```python
from build123d import *

# Parameters (mm, degrees)
ESTRUSIONE_ESTRUSIONE1_DEPTH = 15
SCHIZZO3_W                   = 33
SCHIZZO3_H                   = 6
TAGLIO_ESTRUSIONE1_DEPTH     = 127.609636284
TAGLIO_ESTRUSIONE2_DEPTH     = 127.609636284
FORO_15_0_15_2_D             = 15
FORO_12_0_12_1_D             = 12
SMUSSO1_SIZE                 = 2


with BuildPart() as part:
    # Schizzo2 → Estrusione-Estrusione1 (new, symmetric)
    with BuildSketch(Plane.XY):
        Polygon((0, 0), (123, 0), (123, 13), (115, 13), (115, 26), (30, 26), (30, 20), (0, 20), align=None)
    extrude(amount=ESTRUSIONE_ESTRUSIONE1_DEPTH, both=True)

    # Schizzo3 → Taglio-Estrusione1 (cut, through all)
    with BuildSketch(Plane(origin=(0, 26, 0), x_dir=(1, 0, 0), z_dir=(0, 1, 0))):
        with Locations((106.5, -12)):
            Rectangle(SCHIZZO3_W, SCHIZZO3_H)
        with Locations((106.5, 12)):
            Rectangle(SCHIZZO3_W, SCHIZZO3_H)
    extrude(amount=-TAGLIO_ESTRUSIONE1_DEPTH, mode=Mode.SUBTRACT)

    # Schizzo4 → Taglio-Estrusione2 (cut, through all)
    with BuildSketch(Plane(origin=(0, 26, 0), x_dir=(1, 0, 0), z_dir=(0, 1, 0))):
        with BuildLine():
            Line((45, 5), (75, 5))
            ThreePointArc((75, 5), (80, 0), (75, -5))
            Line((75, -5), (45, -5))
            ThreePointArc((45, -5), (40, 0), (45, 5))
        make_face()
    extrude(amount=-TAGLIO_ESTRUSIONE2_DEPTH, mode=Mode.SUBTRACT)

    # Foro Ø15.0 (15)-2 (through all)
    with Locations(Plane(origin=(0, 20, 0), x_dir=(1, 0, 0), z_dir=(0, 1, 0))):
        with Locations((15, 0)):
            Hole(FORO_15_0_15_2_D / 2)

    # Foro Ø12.0 (12)-1 (through all)
    with Locations(Plane.XY.offset(9)):
        with Locations((102, 12)):
            Hole(FORO_12_0_12_1_D / 2)

    # Smusso1
    smusso1_edges = [part.edges().sort_by_distance(p)[0] for p in [
        (0, 10, -15),
        (0, 10, 15),
    ]]
    chamfer(smusso1_edges, length=SMUSSO1_SIZE)


solid = part.part
```
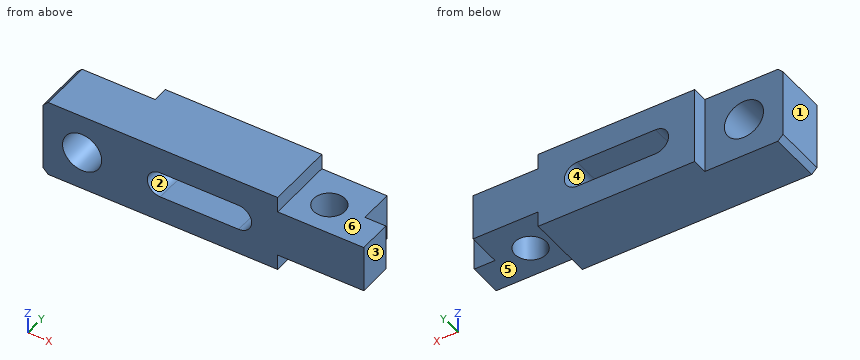
CAD build for the part. Positions are in the model's coordinates, mm. Face numbers are marked on the shaded views. A direction names the side the tool comes from. Round coordinates to 2 decimals unless told otherwise and drop trailing zeros. Order: outer loops, then holes, each group sorted by start corner. A loop starts at its lowest first (then second) coordinate and runs counter-clockwise, first axis right, second up. Notation, with made-up numbers: (82.25, -24.75) - (99.25, -24.75) arc R21 ccw to (99.25, -11.75) - close; hole circle Ø4 at (48, -32.5). An arc over 180 degrees is marked (long way). Answer in a Markdown table with one row per item. Add a question column.
(1) Band-saw the part on B-B on x = 102. List the corners of the cut face in (y, z), and give its area (3 significant figures).
(2) Mould opens along X. For the marked faces 1, 2 and 3 say: +X half, -X half, draft (parallel to the pull), parting line (faces both ways), or undercut.
(3) Band-saw the part on C-C on y = 4.25. List the corners of the cut face in (x, z), and give its area (3 significant figures).
(4) 3-axis set-ups, long thin cutter, end or side, ignore diameter. For the marked faces 4, 5 and 6: which of +Z, -Z, +X, -X, +Y, -Y reach the whole face in a straight line?
(5) Drop flat-ended pins along their axis: pin 1 Ø6.5 at (y, z) = (16.5, -11.5) entering from +X; pin 2 Ø3 at (x, y) = (104.5, 8) entering from +Z; pin 3 Ø2.5 at (x, z) = (118, 2.5) entering from +Y. Give the stop position or say it passes through.
(6) Probe L1, parallel to Y at x = 102, z = -2; L2, parallel to Z at x = 50.5, y = 13; L3, parallel to Z at x = 15, y = 12.25. List the from-to ranges inside material, lowest first. Write a range as [from, to].
(7) Band-saw the part on A-A on z = 0. List the corners of the cut face in (x, y), and give its area (3 significant figures).
(8) Band-saw the part on D-D on x = 62.5. List the corners of the cut face in (y, z), and give its area (3 significant figures).
Data:
| question | item | result |
|---|---|---|
| 1 | outline | (0, -9) - (6, -9) - (6, 9) - (0, 9) - close; (18, -9) - (26, -9) - (26, 9) - (18, 9) - close |
| 1 | area | 252 mm^2 |
| 2 | face 1 | -X half |
| 2 | face 2 | undercut |
| 2 | face 3 | +X half |
| 3 | outline | (0, -13) - (2, -15) - (90, -15) - (90, -9) - (123, -9) - (123, 9) - (90, 9) - (90, 15) - (2, 15) - (0, 13) - close; hole circle Ø15 at (15, 0); hole (45, -5) - (75, -5) arc R5 ccw to (75, 5) - (45, 5) arc R5 ccw to start |
| 3 | area | 2,730 mm^2 |
| 4 | face 4 | +Y, -Y |
| 4 | face 5 | -Z, +X, +Y, -Y |
| 4 | face 6 | +Z, +X, +Y, -Y |
| 5 | pin 1 | stops at x = 115 |
| 5 | pin 2 | stops at z = 9 |
| 5 | pin 3 | stops at y = 13 |
| 6 | L1 | y = [0, 6], [18, 26] |
| 6 | L2 | z = [-15, -5], [5, 15] |
| 6 | L3 | z = [-15, -7.5], [7.5, 15] |
| 7 | outline | (0, 0) - (7.5, 0) - (7.5, 20) - (0, 20) - close; (22.5, 0) - (40, 0) - (40, 26) - (30, 26) - (30, 20) - (22.5, 20) - close; (80, 0) - (123, 0) - (123, 13) - (115, 13) - (115, 26) - (80, 26) - close; hole circle Ø12 at (102, 12) |
| 7 | area | 1,460 mm^2 |
| 8 | outline | (0, -15) - (26, -15) - (26, -5) - (0, -5) - close; (0, 5) - (26, 5) - (26, 15) - (0, 15) - close |
| 8 | area | 520 mm^2 |
